Geometry: see drawing. Coordinates: mm, zero at the bounding-box minimum. A direction names the side the tool comes from. Round coordinates to 2 decimals unless told otherwise and drop trailing zeros. Loops run counter-clockwise (first coordinate to the right, second up) from the corner with the lowest first, then second, coordinate; pieces in that order, holes last. Notation, with made-up numbers: (63, 17) -> (99, 17) arc R12 ccw to (99, 32) -> close; hole circle Ø2 at (-16, 89.5). An arc over 180 degrees is marked (long way). Answer in a Markdown table with one row per item.
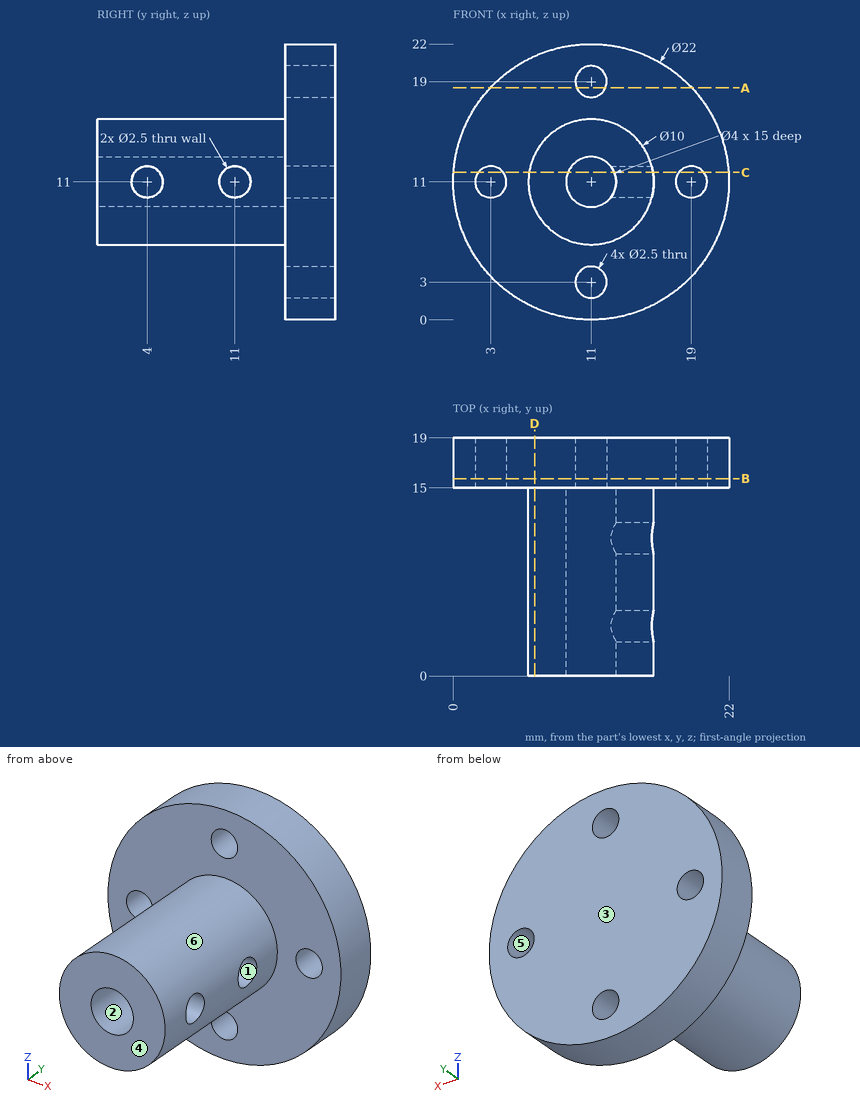
Item 1: Set-up query: the marked faces 1, 2 and 3. Return all of +Z, -Z, +X, -X, +Y, -Y with unobstructed straight access to the full face (end or side cutting, diameter ignored); none if empty.
Ans:
| item | result |
|---|---|
| face 1 | +X |
| face 2 | -Y |
| face 3 | +Z, -Z, +X, -X, +Y |
Item 2: Section query A-A, the plane z = 18.5. Output: boundary loops of the cut face in (x, y), and give its area (3 significant figures).
Ans:
| item | result |
|---|---|
| outline | (2.95, 15) -> (9.85, 15) -> (9.85, 19) -> (2.95, 19) -> close; (12.15, 15) -> (19.05, 15) -> (19.05, 19) -> (12.15, 19) -> close |
| area | 55.2 mm2 |
Item 3: Ray query, L1, parallel to Y at x = 14.5, z = 11; L2, parallel to X at y = 16.85, z = 11; L3, parallel to Y at x = 5, z = 13.5. Return the intervals inside material, ascending.
Ans:
| item | result |
|---|---|
| L1 | 0 to 2.75, 5.25 to 9.75, 12.25 to 19 |
| L2 | 0 to 1.75, 4.25 to 17.75, 20.25 to 22 |
| L3 | 15 to 19 |
Item 4: First-contact query: P1, Ø3, axis at x = 11, z = 3, coming from the +Y side; P2, Ø5, axis at x = 8.5, y = 14, coming from the -Z side; P3, Ø2, axis at x = 18.5, y = 15, coming from the -Z side; P4, Ø2, axis at x = 13, z = 17.5, coming from the -Y side. Flat tips, straight axial feed; report the tip coordinate or a pass-through.
Ans:
| item | result |
|---|---|
| P1 | y = 19 |
| P2 | z = 0 |
| P3 | z = 2.13 |
| P4 | y = 15 |
Item 5: Section query D-D, the plane x = 6.5. Output: boundary loops of the cut face in (y, z), and give its area (3 significant figures).
Ans:
| item | result |
|---|---|
| outline | (0, 8.82) -> (15, 8.82) -> (15, 0.96) -> (19, 0.96) -> (19, 21.04) -> (15, 21.04) -> (15, 13.18) -> (0, 13.18) -> close |
| area | 146 mm2 |
Item 6: Mould query, pull axis Z, two halves, no side actions, for the marked faces 4, 5 and 6. Classes: released by +Z, released by -Z, zero draft, split by the parting line, or undercut.
Ans:
| item | result |
|---|---|
| face 4 | zero draft |
| face 5 | undercut |
| face 6 | split by the parting line |
Item 7: Section query C-C, the plane z = 11.75. Output: boundary loops of the cut face in (x, y).
Ans:
| item | result |
|---|---|
| outline | (0.03, 15) -> (2, 15) -> (2, 19) -> (0.03, 19) -> close; (4, 15) -> (6.06, 15) -> (6.06, 0) -> (9.15, 0) -> (9.15, 15) -> (12.85, 15) -> (12.85, 12) -> (15.94, 12) -> (15.94, 15) -> (18, 15) -> (18, 19) -> (4, 19) -> close; (12.85, 0) -> (15.94, 0) -> (15.94, 3) -> (12.85, 3) -> close; (12.85, 5) -> (15.94, 5) -> (15.94, 10) -> (12.85, 10) -> close; (20, 15) -> (21.97, 15) -> (21.97, 19) -> (20, 19) -> close |
Item 8: Section query B-B, the plane y = 15.75. Output: boundary loops of the cut face in (x, z).
Ans:
| item | result |
|---|---|
| outline | circle Ø22 at (11, 11); hole circle Ø2.5 at (3, 11); hole circle Ø2.5 at (11, 3); hole circle Ø2.5 at (11, 19); hole circle Ø2.5 at (19, 11) |
